Design review of the part built by this model. Coordinates are the model's own, in mm. A direction names the side the tool comes from. Give positions to 0.01 mm unless a question says otherwise; leave off trailing zeros. Order: outer loops, then holes, each group sorted by start corner. A loop starts at its lowest first (then second) coordinate and runs counter-clockwise, first axis right, second up. Notation, with made-up numbers: (5, 83) -> (44, 83) arc R17 ccw to (44, 97) -> close; hole circle Ø5 at (-33, -13). An arc over 180 degrees is marked (long way). Return JSON: item names as keys, results as strings.
```python
from build123d import *

# Parameters (mm, degrees)
F0_R       = 5.8934645996
F1_DEPTH   = 25.4
F4_D       = 12.7
F4_ON_F3_D = 12.7
F5_SIZE    = 6.35


with BuildPart() as f1:
    # F0 (on Top) → F1 (new body)
    with BuildSketch(Plane.XY):
        with BuildLine():
            ThreePointArc((23.6362737938, 28.2139556626), (14.1364445597, 16.9249221875), (0, 12.7))
            Line((0, 12.7), (-76.2, 12.7))
            Line((-76.2, 12.7), (-76.2, -12.7))
            Line((-76.2, -12.7), (0, -12.7))
            ThreePointArc((0, -12.7), (9.3073343437, -15.5213038758), (15.4816922387, -23.0355259068))
            ThreePointArc((15.4816922387, -23.0355259068), (24.8374177204, -34.4214869615), (38.9404008269, -38.6964812219))
            Line((38.9404008269, -38.6964812219), (115.1404008269, -38.6964812219))
            Line((115.1404008269, -38.6964812219), (115.1404008269, -13.2964812219))
            Line((115.1404008269, -13.2964812219), (38.9404008269, -13.2964812219))
            ThreePointArc((38.9404008269, -13.2964812219), (26.9165705995, -0.2651159667), (39.6211307376, 12.1035187781))
            Line((39.6211307376, 12.1035187781), (115.8211307376, 12.1035187781))
            Line((115.8211307376, 12.1035187781), (115.8211307376, 37.5035187781))
            Line((115.8211307376, 37.5035187781), (33.2611742348, 37.5035187781))
            ThreePointArc((33.2611742348, 37.5035187781), (27.5216816712, 33.819244205), (23.6362737938, 28.2139556626))
        make_face()
        with Locations((-63.5, 0)):
            Circle(F0_R, mode=Mode.SUBTRACT)
    extrude(amount=F1_DEPTH)

    # F4 (through all)
    with Locations(Plane.XZ.offset(38.6964812219)):
        with Locations((97.5403962757, 12.6839925341)):
            Hole(F4_D / 2)

    # F4 on F3 (through all)
    with Locations(Plane(origin=(0, 37.5035187781, 0), x_dir=(-1, 0, 0), z_dir=(0, 1, 0))):
        with Locations((-97.8747204662, 12.5663767254)):
            Hole(F4_ON_F3_D / 2)

    # F5
    f5_edges = [f1.edges().sort_by_distance(p)[0] for p in [
        (115.140401, -25.996481, 25.4),
        (115.140401, -25.996481, 0),
        (115.821131, 24.803519, 25.4),
        (115.821131, 24.803519, 0),
    ]]
    chamfer(f5_edges, length=F5_SIZE)


solid = f1.part
```
Item 1: Wall thickness on L1, parallel to Y at x = 95, z = 20.25; L2, parallel to Y at x = -63.5, z = 6; L3, parallel to Z at x = 98, y = -22.5: over which ranges is each line inside the solid? List them lowest first. Write a range as [from, to].
Result set:
{"L1": "y = [-38.7, -13.3], [12.1, 37.5]", "L2": "y = [-12.7, -5.89], [5.89, 12.7]", "L3": "z = [0, 6.22], [19.02, 25.4]"}
Item 2: Add section D-D (y = -34). Give the boundary of the cut face in (x, z).
Result set:
{"outline": "(24.23, 0) -> (108.79, 0) -> (115.14, 6.35) -> (115.14, 19.05) -> (108.79, 25.4) -> (24.23, 25.4) -> close; hole (95.6, 6.64) arc R6.35 ccw (long way) to (99.81, 18.61) arc R6.35 ccw (long way) to start"}
Item 3: Machinability: for faces 4 (the face through (-39, -12.7, 13)), 5 (the face through (115.14, -26, 13)), 6 (the face through (78, -13.296, 13)), which of the approach directions +Z, -Z, +X, -X, +Y, -Y give a long, thin tool a straight path to every point of the face, cutting with its end or side? Answer none if there is none.
Result set:
{"face 4": "+Z, -Z, -X, -Y", "face 5": "+Z, -Z, +X, -Y", "face 6": "+Z, -Z, +X"}
Item 4: Mouldability with a two-part tool opening along X and no side actions: class faces 1 (the face through (9.192, -15.445, 12.522)), 2 (the face through (103.82, 24.63, 10.33)), 3 (the face through (112.69, 24.63, 22.18)) as released by +X, released by -X, zero draft, split by the parting line, or undercut.
Result set:
{"face 1": "released by -X", "face 2": "undercut", "face 3": "released by +X"}
Item 5: Add section A-A (z = 16.5). Give the boundary of the cut face in (x, y).
Result set:
{"outline": "(-76.2, -12.7) -> (0, -12.7) arc R16.76 cw to (15.48, -23.04) arc R25.4 ccw to (38.94, -38.7) -> (92.46, -38.7) -> (92.46, -13.3) -> (38.94, -13.3) arc R12.71 cw to (39.62, 12.1) -> (92.46, 12.1) -> (92.46, 37.5) -> (33.26, 37.5) arc R17.42 ccw to (23.64, 28.21) arc R25.76 cw to (0, 12.7) -> (-76.2, 12.7) -> close; (102.86, -38.7) -> (115.14, -38.7) -> (115.14, -13.3) -> (102.86, -13.3) -> close; (102.86, 12.1) -> (115.82, 12.1) -> (115.82, 37.5) -> (102.86, 37.5) -> close; hole circle Ø11.79 at (-63.5, 0)"}
Item 6: Add section B-B (x = -63.5). Give the boundary of the cut face in (y, z).
Result set:
{"outline": "(-12.7, 0) -> (-5.89, 0) -> (-5.89, 25.4) -> (-12.7, 25.4) -> close; (5.89, 0) -> (12.7, 0) -> (12.7, 25.4) -> (5.89, 25.4) -> close"}
Item 7: For pin 1 (2 mm diameter, centred on x = -27.5, z = 22.5, fed in from -Y); pin 2 (2 mm diameter, centred on y = -26.5, z = 8.5, fed in from -X); pin 3 (6.5 mm diameter, centred on y = -23.5, z = 12, fed in from +X), all flat-tipped, find the tip position at first contact; note any pin that passes through.
Result set:
{"pin 1": "stops at y = -12.7", "pin 2": "stops at x = 16.66", "pin 3": "stops at x = 115.14"}
Item 8: Add section C-C (y = 3.5). Give the boundary of the cut face in (x, z).
Result set:
{"outline": "(-76.2, 0) -> (-68.24, 0) -> (-68.24, 25.4) -> (-76.2, 25.4) -> close; (-58.76, 0) -> (27.59, 0) -> (27.59, 25.4) -> (-58.76, 25.4) -> close"}
